The model under review builds one solid part; all positions refer to its coordinate system, in mm. Face numbers are marked on the shaded views. A direction names the side the tool comes from. Give positions to 0.01 mm unless a question says otherwise; leave off trailing zeros. Write each loop counter-clockwise with the first axis right and the second up, starting at its lowest first coordinate (ties: lowest second). Pieces come first, ordered by that corner, then holes.
from build123d import *

# Parameters (mm, degrees)
BOSS_EXTRUDE1_DEPTH = 50
SKETCH2_R           = 11
SKETCH2_R_2         = 1.5
CUT_EXTRUDE1_DEPTH  = 2
CUT_EXTRUDE2_DEPTH  = 2
CUT_EXTRUDE3_DEPTH  = 2
CUT_EXTRUDE4_DEPTH  = 2


with BuildPart() as part:
    # Sketch1 → Boss-Extrude1 (new body)
    with BuildSketch(Plane(origin=(0, 0, 0), x_dir=(0, 0, -1), z_dir=(1, 0, 0))):
        with BuildLine():
            Line((4, 0), (53, 0))
            Line((53, 0), (53, 2))
            Line((53, 2), (4, 2))
            ThreePointArc((4, 2), (2.585786438, 2.585786438), (2, 4))
            Line((2, 4), (2, 51))
            Line((2, 51), (0, 51))
            Line((0, 51), (0, 4))
            ThreePointArc((0, 4), (1.171572875, 1.171572875), (4, 0))
        make_face()
    extrude(amount=BOSS_EXTRUDE1_DEPTH)

    # Sketch2 → Cut-Extrude1 (cut)
    with BuildSketch(Plane(origin=(0, 0, -2), x_dir=(-1, 0, 0), z_dir=(0, 0, -1))):
        with Locations((-25, 30)):
            Circle(SKETCH2_R)
        with Locations((-9.5, 45.5)):
            Circle(SKETCH2_R_2)
        with Locations((-40.488, 45.5)):
            Circle(SKETCH2_R_2)
        with Locations((-40.488, 14.5)):
            Circle(SKETCH2_R_2)
        with Locations((-9.5, 14.5)):
            Circle(SKETCH2_R_2)
    extrude(amount=-CUT_EXTRUDE1_DEPTH, mode=Mode.SUBTRACT)

    # Sketch3 → Cut-Extrude2 (cut)
    with BuildSketch(Plane(origin=(0, 2, 0), x_dir=(1, 0, 0), z_dir=(0, 1, 0))):
        with BuildLine():
            Line((42.1, 42), (42.1, 12))
            ThreePointArc((42.1, 12), (40, 9.9), (37.9, 12))
            Line((37.9, 12), (37.9, 42))
            ThreePointArc((37.9, 42), (40, 44.1), (42.1, 42))
        make_face()
        with BuildLine():
            Line((7.9, 42), (7.9, 12))
            ThreePointArc((7.9, 12), (10, 9.9), (12.1, 12))
            Line((12.1, 12), (12.1, 42))
            ThreePointArc((12.1, 42), (10, 44.1), (7.9, 42))
        make_face()
    extrude(amount=-CUT_EXTRUDE2_DEPTH, mode=Mode.SUBTRACT)

    # Sketch4 → Cut-Extrude3 (cut)
    with BuildSketch(Plane(origin=(0, 2, 0), x_dir=(1, 0, 0), z_dir=(0, 1, 0))):
        Polygon((0, 53), (0, 43), (10, 53), align=None)
        Polygon((50, 53), (40, 53), (50, 43), align=None)
    extrude(amount=-CUT_EXTRUDE3_DEPTH, mode=Mode.SUBTRACT)

    # Sketch5 → Cut-Extrude4 (cut)
    with BuildSketch(Plane(origin=(0, 0, -2), x_dir=(-1, 0, 0), z_dir=(0, 0, -1))):
        Polygon((-50, 41), (-40, 51), (-50, 51), align=None)
        Polygon((-10, 51), (0, 41), (0, 51), align=None)
    extrude(amount=-CUT_EXTRUDE4_DEPTH, mode=Mode.SUBTRACT)


solid = part.part
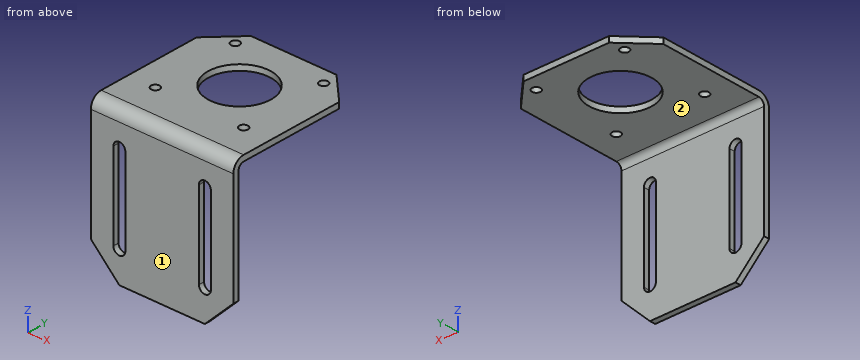
1) Insertion check: pin 1 (23.5 mm diameter, centred on x = 29.5, y = 35.5, fed in from -Z); pin 2 (24.5 mm diameter, centred on x = 20.5, z = -21, fed in from +Y). Each pin has a flat end and moves straight along its axis. Give the tip position at first contact, or say it passes through.
2) Consider section A-A, the plane x = 25. Give the boundary of the cut face in (y, z), then the cut area to 3 significant figures.
3) Tool access review of the marked faces 1 and 2: name each direction out of +Z, -Z, +X, -X, +Y, -Y from which nothing blocks a thin tool from reaching the whole face with its end or side.
4) Consider section B-B, the plane y = 14.5. Give the boundary of the cut face in (x, z), then the cut area to 3 significant figures.
5) Consider section C-C, the plane z = -31.5. Give the boundary of the cut face in (x, y), then the cut area to 3 significant figures.
6) Consider section D-D, the plane y = 35. Give the boundary of the cut face in (x, z).
7) To check wall thickness, follow probe 1 along Y at (x, z) = (9.5, -1.3); probe 2 along Z at (x, y) = (11, 6); probe 3 along Y at (x, z) = (20, -38.5). State the ranges of each line that lie inside material, in increasing order.
Answer block:
1. pin 1: stops at z = -2
1. pin 2: stops at y = 2
2. outline: (0, -53) - (2, -53) - (2, -4) arc R2 cw to (4, -2) - (19, -2) - (19, 0) - (4, 0) arc R4 ccw to (0, -4) - close; (41, -2) - (51, -2) - (51, 0) - (41, 0) - close
2. area: 157 mm2
3. face 1: +Z, -Z, +X, -X, -Y
3. face 2: -Z, +X, -X, +Y
4. outline: (0, -2) - (8, -2) - (8, 0) - (0, 0) - close; (11, -2) - (38.99, -2) - (38.99, 0) - (11, 0) - close; (41.99, -2) - (50, -2) - (50, 0) - (41.99, 0) - close
4. area: 88.0 mm2
5. outline: (0, 0) - (7.9, 0) - (7.9, 2) - (0, 2) - close; (12.1, 0) - (37.9, 0) - (37.9, 2) - (12.1, 2) - close; (42.1, 0) - (50, 0) - (50, 2) - (42.1, 2) - close
5. area: 83.2 mm2
6. outline: (0, -2) - (15.2, -2) - (15.2, 0) - (0, 0) - close; (34.8, -2) - (50, -2) - (50, 0) - (34.8, 0) - close
7. probe 1: y = 1.05 to 13, 16 to 44, 47 to 50.5
7. probe 2: z = -2 to 0
7. probe 3: y = 0 to 2
